Here's how the part is built. I have some questions about the finished solid (model axes, mm). A direction names the side the tool comes from. Round coordinates to 2 decimals unless told otherwise and drop trailing zeros. Write each loop counter-clockwise with the first axis right and the second up, starting at its lowest first coordinate (ties: lowest second). Pieces come first, ordered by that corner, then holes. Notation, with made-up numbers: (-27, -26.75) -> (29, -26.75) arc R13 ccw to (29, -17.75) -> close; hole circle Ø3 at (89, 38.25). An arc over 180 degrees is marked (long way). Answer as CSV lines item,"result".
```python
from build123d import *

# Parameters (mm, degrees)
F0_W     = 76.2
F0_H     = 79.375
F1_DEPTH = 3.81
F2_W     = 63.5
F2_H     = 76.2
F3_DEPTH = 1.905
F4_W     = 6.35
F4_H     = 50.8
F5_DEPTH = 25.4
F7_DEPTH = 25.4
F8_W     = 50.8
F8_H     = 5.08
F9_DEPTH = 25.4


with BuildPart() as f1:
    # F0 (on Top) → F1 (new body)
    with BuildSketch(Plane.XY):
        Rectangle(F0_W, F0_H)
    extrude(amount=F1_DEPTH)

    # F2 (on face) → F3 (cut)
    with BuildSketch(Plane.XY.offset(3.81)):
        Rectangle(F2_W, F2_H)
    extrude(amount=-F3_DEPTH, mode=Mode.SUBTRACT)

    # F4 (on face) → F5 (join)
    with BuildSketch(Plane.XY.offset(1.905)):
        Rectangle(F4_W, F4_H)
    extrude(amount=F5_DEPTH)

    # F6 (on face) → F7 (cut)
    with BuildSketch(Plane.YZ.offset(3.175)):
        with BuildLine():
            ThreePointArc((15.24, 9.525), (20.32, 14.605), (15.24, 19.685))
            Line((15.24, 19.685), (-15.24, 19.685))
            ThreePointArc((-15.24, 19.685), (-20.32, 14.605), (-15.24, 9.525))
            Line((-15.24, 9.525), (15.24, 9.525))
        make_face()
    extrude(amount=-F7_DEPTH, mode=Mode.SUBTRACT)

    # F8 (on face) → F9 (cut)
    with BuildSketch(Plane.YZ.offset(3.175)):
        with Locations((0, 24.765)):
            Rectangle(F8_W, F8_H)
    extrude(amount=-F9_DEPTH, mode=Mode.SUBTRACT)


solid = f1.part
```
1. For pin 1 Ø10 at (x, y) = (25, 0.5) entering from +Z (3 decimals); pin 2 Ø7 at (x, z) = (1.5, 10.5) entering from -Y; pin 3 Ø10 at (y, z) = (14, 9.5) entering from +X (3 decimals), each with a flat end and sliding along its axis, tell me the tip position at first contact or that it passes through.
Numbers:
pin 1,"stops at z = 1.905"
pin 2,"stops at y = -25.4"
pin 3,"stops at x = 3.175"
2. Suppose I cut it at C-C on y = -30. Please give me the cut outline in (x, z) (3 decimals), and give its area (3 significant figures).
Numbers:
outline,"(-38.1, 0) -> (38.1, 0) -> (38.1, 3.81) -> (31.75, 3.81) -> (31.75, 1.905) -> (-31.75, 1.905) -> (-31.75, 3.81) -> (-38.1, 3.81) -> close"
area,"169 mm^2"
3. If I drill on line 1 (Y direction, x = 5, z = 3); line 2 (X direction, y = -4.5, z = 2.75) (3 decimals); line 3 (Z direction, x = 30, y = 31) (3 decimals), over which ranges is the centre line in solid material (lowest first)?
Numbers:
line 1,"y = -39.69 to -38.1, 38.1 to 39.69"
line 2,"x = -38.1 to -31.75, -3.175 to 3.175, 31.75 to 38.1"
line 3,"z = 0 to 1.905"
4. If we mould it in two halves opening along X, with no side actions, what happens to faces 1 (the face through (38.1, -1, 2)), 2 (the face through (0, 38.1, 3)), 3 (the face through (-0.2, 38.4, 3.81))? For each: released by +X, released by -X, zero draft, split by the parting line, or undercut.
Numbers:
face 1,"released by +X"
face 2,"undercut"
face 3,"zero draft"
5. On a 3-axis mill with a long thin cutter (end or side, diameter ignored), from which of +Z, -Z, +X, -X, +Y, -Y can I reach the whole of each face in a straight line? I mean faces 4 (the face through (0, -38.1, 3)), 5 (the face through (0.04, -20.32, 14.72)), 6 (the face through (0, 0, 22.225)). Say none if no direction works.
Numbers:
face 4,"+Z"
face 5,"+X, -X"
face 6,"+Z, +X, -X, +Y, -Y"
6. Suppose I cut it at B-B on z = 16.5. Please give me the cut outline in (x, y) (3 decimals).
Numbers:
outline,"(-3.175, -25.4) -> (3.175, -25.4) -> (3.175, -19.953) -> (-3.175, -19.953) -> close; (-3.175, 19.953) -> (3.175, 19.953) -> (3.175, 25.4) -> (-3.175, 25.4) -> close"
7. Suppose I cut it at A-A on y = -8. Please give me the cut outline in (x, z) (3 decimals), and give its area (3 significant figures).
Numbers:
outline,"(-38.1, 0) -> (38.1, 0) -> (38.1, 3.81) -> (31.75, 3.81) -> (31.75, 1.905) -> (3.175, 1.905) -> (3.175, 9.525) -> (-3.175, 9.525) -> (-3.175, 1.905) -> (-31.75, 1.905) -> (-31.75, 3.81) -> (-38.1, 3.81) -> close; (-3.175, 19.685) -> (3.175, 19.685) -> (3.175, 22.225) -> (-3.175, 22.225) -> close"
area,"234 mm^2"
